Verification items for the finished model (mm, model axes). Face numbers are marked on the shaded views. A direction names the side the tool comes from. Coordinates: 2 decimals unless noted, no trailing zeros. Order: outer loops, then holes, each group sorted by start corner. A loop starts at its lowest first (then second) coordinate and runs counter-clockwise, first axis right, second up. Notation, with made-up numbers: M -5,26 L 51,26 A16 cw 51,57 Z; hole C 48,47 d2. An arc over 180 degrees is marked long. Return JSON: item names as keys, results as strings. Group by question number.
1. Gauge pin test, flat ends, axial feed: pin 1 (8 mm diameter, centred on x = 2.5, z = -1, fed in from -Y); pin 2 (2 mm diameter, centred on x = 0, y = 2, fed in from -Z). Record the tip position at first contact, or that the pin passes through.
2. Set-up check for the marked faces 4 and 5: record each of +Z, -Z, +X, -X, +Y, -Y from which the full face is reachable in a straight line by a thin tool's end or side.
3. Material ranges on line 1 along X through (y, z) = (2.6, -5.25); line 2 along Z through (x, y) = (1, 3.1); line 3 along Z through (x, y) = (-3.25, 3.15), recorded low to high.
4. Section check B-B, the plane y = 1.85. Record the cut outline in (x, z), plus the area to 4 significant figures.
5. Section check C-C, the plane x = -0.75. Record the cut outline in (y, z), plus the area to 3 significant figures.
6. Mould release check, pull along X, two halves, no side actions. Record for the marked faces 1, 2 and 3: +X half, -X half, draft (parallel to the pull), parting line (faces both ways), or undercut.
7. Section check A-A, the plane z = -11.75. Record the cut outline in (x, y), plus the area to 3 significant figures.
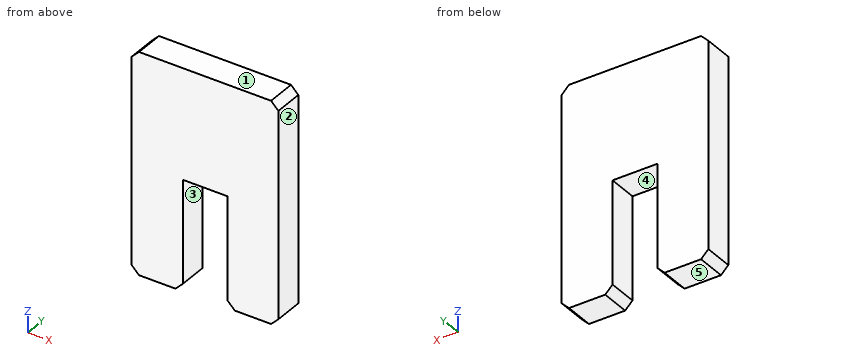
```python
from build123d import *

# Parameters (mm, degrees)
SKIZZE1_W                       = 20
SKIZZE1_H                       = 30
AUFSATZ_LINEAR_AUSTRAGEN1_DEPTH = 4
SKIZZE2_W                       = 6.1
SKIZZE2_H                       = 15
SCHNITT_LINEAR_AUSTRAGEN1_DEPTH = 5
FASE1_SIZE                      = 1


with BuildPart() as part:
    # Skizze1 → Aufsatz-Linear austragen1 (new body)
    with BuildSketch(Plane(origin=(0, 0, 0), x_dir=(1, 0, 0), z_dir=(0, 1, 0))):
        Rectangle(SKIZZE1_W, SKIZZE1_H)
    extrude(amount=AUFSATZ_LINEAR_AUSTRAGEN1_DEPTH)

    # Skizze2 → Schnitt-Linear austragen1 (cut, through all)
    with BuildSketch(Plane(origin=(0, 4, 0), x_dir=(1, 0, 0), z_dir=(0, 1, 0))):
        with Locations((0.014627906, 7.5)):
            Rectangle(SKIZZE2_W, SKIZZE2_H)
    extrude(amount=-SCHNITT_LINEAR_AUSTRAGEN1_DEPTH, mode=Mode.SUBTRACT)

    # Fase1
    fase1_edges = [part.edges().sort_by_distance(p)[0] for p in [
        (-3.035372094, 2, -15),
        (3.064627906, 2, -15),
        (10, 2, 15),
        (-10, 2, 15),
        (-10, 2, -15),
        (10, 2, -15),
    ]]
    chamfer(fase1_edges, length=FASE1_SIZE)


solid = part.part
```
Answers follow:
{
 "1": {"pin 1": "y = 0", "pin 2": "z = 0"},
 "2": {"face 4": "-Z, +Y, -Y", "face 5": "-Z, +X, -X, +Y, -Y"},
 "3": {"line 1": "-10 to -3.04, 3.06 to 10", "line 2": "0 to 15", "line 3": "-14.21 to 15"},
 "4": {"outline": "M -10,-14 L -9,-15 L -4.04,-15 L -3.04,-14 L -3.04,0 L 3.06,0 L 3.06,-14 L 4.06,-15 L 9,-15 L 10,-14 L 10,14 L 9,15 L -9,15 L -10,14 Z", "area": "505.5 mm^2"},
 "5": {"outline": "M 0,0 L 4,0 L 4,15 L 0,15 Z", "area": "60.0 mm^2"},
 "6": {"face 1": "draft", "face 2": "+X half", "face 3": "undercut"},
 "7": {"outline": "M -10,0 L -3.04,0 L -3.04,4 L -10,4 Z; M 3.06,0 L 10,0 L 10,4 L 3.06,4 Z", "area": "55.6 mm^2"}
}
